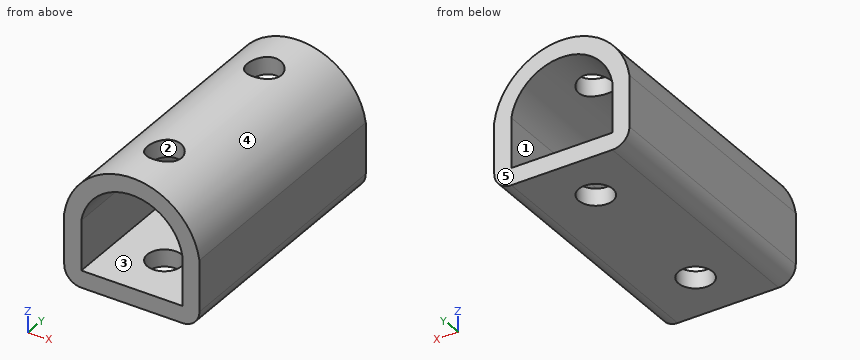
```python
from build123d import *

# Parameters (mm, degrees)
F1_DEPTH = 75
F3_DEPTH = 75.001
F4_R     = 5
F5_DEPTH = 37.1620739384
F6_R     = 5


# Not quite as in the source:
# - a feature of the source that left no trace in its solid (it failed there, or was rolled back) is left out


with BuildPart() as f1:
    # F0 (on Front) → F1 (new body)
    with BuildSketch(Plane.XZ):
        with BuildLine():
            ThreePointArc((39.5949743688, 20), (19.7974871844, 37.1610739384), (0, 20))
            Line((0, 20), (0, 0))
            Line((0, 0), (39.5949743688, 0))
            Line((39.5949743688, 0), (39.5949743688, 20))
        make_face()
    extrude(amount=F1_DEPTH)

    # F2 (on face) → F3 (cut, through all)
    with BuildSketch(Plane.XZ.offset(75)):
        with BuildLine():
            Line((34.5949743688, 5), (34.5949743688, 19.6175700258))
            ThreePointArc((34.5949743688, 19.6175700258), (19.7974871844, 32.1610739384), (5, 19.6175700258))
            Line((5, 19.6175700258), (5, 5))
            Line((5, 5), (34.5949743688, 5))
        make_face()
    extrude(amount=-F3_DEPTH, mode=Mode.SUBTRACT)

    # F4 (on face) → F5 (cut, through all)
    with BuildSketch(Plane(origin=(0, 0, 0), x_dir=(1, 0, 0), z_dir=(0, 0, -1))):
        with Locations((19.5949743688, 60)):
            Circle(F4_R)
        with Locations((19.5949743688, 15)):
            Circle(F4_R)
    extrude(amount=-F5_DEPTH, mode=Mode.SUBTRACT)

    # F6
    f6_edges = [f1.edges().sort_by_distance(p)[0] for p in [
        (39.594974, -37.5, 0),
        (0, -37.5, 0),
    ]]
    fillet(f6_edges, radius=F6_R)


solid = f1.part
```
Here's how the part is built. I have some questions about the finished solid (model axes, mm). Face numbers are marked on the shaded views. A direction names the side the tool comes from. Give positions to 0.01 mm unless a question says otherwise; leave off trailing zeros. Write each loop counter-clockwise with the first axis right and the second up, starting at its lowest first coordinate (ties: lowest second). Pieces come first, ordered by that corner, then holes. Notation, with made-up numbers: (72, 73) -> (114, 73) arc R11 ccw to (114, 92) -> close; hole circle Ø2 at (82.5, -38.75). An arc over 180 degrees is marked (long way). Use one line per item in the form item = value.
1) Suppose I cut it at C-C (x = 28). Please give me the cut outline in (y, z), and give its area (3 significant figures).
Verdict:
outline = (-75, 0) -> (0, 0) -> (0, 5) -> (-75, 5) -> close; (-75, 29.72) -> (0, 29.72) -> (0, 35.4) -> (-75, 35.4) -> close
area = 801 mm2
2) We'd pull the mould along X, two halves only. Please class the marked faces 3, 4 and 5: +X half, -X half, draft (parallel to the pull), parting line (faces both ways), or undercut.
Verdict:
face_3 = undercut
face_4 = parting line
face_5 = draft
3) I'm going to push flat-ended pins straight in: pin 1 (2 mm diameter, centred on y = -17, z = 33, fed in from -X); pin 2 (5 mm diameter, centred on x = 8.5, y = -20, fed in from +Z); pin 3 (1.5 mm diameter, centred on x = 22, y = -14, fed in from +Z). Where does each tip first touch, or does it pass through?
Verdict:
pin_1 = 6.39
pin_2 = 35.12
pin_3 = through
4) If I drill on L1, parallel to X at y = -52.5, z = 14; L2, parallel to X at y = -15, z = 33; L3, parallel to Z at x = 10, y = -11, over which ranges is the centre line in solid material (lowest first)? Write a range as [from, to].
Verdict:
L1 = [0, 5], [34.59, 39.59]
L2 = [7.59, 14.59], [24.59, 32.01]
L3 = [0, 5], [28.52, 34.6]
5) Suppose I cut it at B-B (y = -68). Please give me the cut outline in (x, z), and give its area (3 significant figures).
Verdict:
outline = (0, 5) arc R5 ccw to (5, 0) -> (34.59, 0) arc R5 ccw to (39.59, 5) -> (39.59, 20) arc R20 ccw to (0, 20) -> close; hole (5, 5) -> (34.59, 5) -> (34.59, 19.62) arc R15 ccw to (5, 19.62) -> close
area = 584 mm2
6) On a 3-axis mill with a long thin cutter (end or side, diameter ignored), from which of +Z, -Z, +X, -X, +Y, -Y can I reach the whole of each face in a straight line? I mean the marked faces 1 and 2. Say none if no direction works.
Verdict:
face_1 = +Y, -Y
face_2 = +Z, -Z
7) Suppose I cut it at A-A (z = 13). Please give me the cut outline in (x, y), and give its area (3 significant figures).
Verdict:
outline = (0, -75) -> (5, -75) -> (5, 0) -> (0, 0) -> close; (34.59, -75) -> (39.59, -75) -> (39.59, 0) -> (34.59, 0) -> close
area = 750 mm2
8) Suppose I cut it at D-D (y = -60). Please give me the cut outline in (x, z).
Verdict:
outline = (0, 5) arc R5 ccw to (5, 0) -> (14.59, 0) -> (14.59, 5) -> (5, 5) -> (5, 19.62) arc R15 cw to (14.59, 31.23) -> (14.59, 36.47) arc R20 ccw to (0, 20) -> close; (24.59, 0) -> (34.59, 0) arc R5 ccw to (39.59, 5) -> (39.59, 20) arc R20 ccw to (24.59, 36.58) -> (24.59, 31.37) arc R15 cw to (34.59, 19.62) -> (34.59, 5) -> (24.59, 5) -> close
